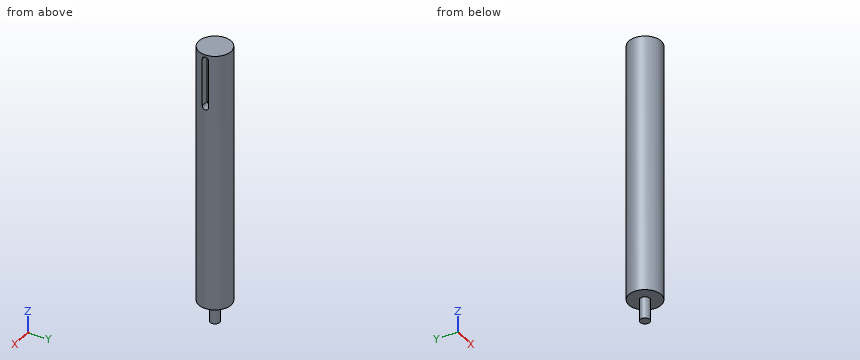
```python
from build123d import *

# Parameters (mm, degrees)
SKETCH_1_R          = 15
EXTRUDE_1_DEPTH     = 240
SKETCH_4_R          = 4.5
EXTRUDE_2_DEPTH     = 20
CUT_EXTRUDE_3_DEPTH = 8


with BuildPart() as part:
    # 草图1 → 凸台-拉伸1 (new body)
    with BuildSketch(Plane.XY):
        Circle(SKETCH_1_R)
    extrude(amount=EXTRUDE_1_DEPTH)

    # 草图4 → 凸台-拉伸2 (add)
    with BuildSketch(Plane(origin=(0, 0, 0), x_dir=(-1, 0, 0), z_dir=(0, 0, -1))):
        Circle(SKETCH_4_R)
    extrude(amount=EXTRUDE_2_DEPTH)

    # 草图5 → 切除-拉伸3 (cut)
    with BuildSketch(Plane(origin=(15, 0, 0), x_dir=(0, 0, -1), z_dir=(1, 0, 0))):
        with BuildLine():
            Line((-235, 3), (-191, 3))
            ThreePointArc((-191, 3), (-188, 0), (-191, -3))
            Line((-191, -3), (-235, -3))
            ThreePointArc((-235, -3), (-238, 0), (-235, 3))
        make_face()
    extrude(amount=-CUT_EXTRUDE_3_DEPTH, mode=Mode.SUBTRACT)


solid = part.part
```
The model under review builds one solid part; all positions refer to its coordinate system, in mm. Round coordinates to 2 decimals unless told otherwise and drop trailing zeros. Write each loop counter-clockwise with the first axis right and the second up, starting at its lowest first coordinate (ties: lowest second). Pieces come first, ordered by that corner, then holes. Notation, with made-up numbers: (-5.75, 35.5) - (38.25, 35.5) arc R17 ccw to (38.25, 66.5) - close; hole circle Ø3 at (-16.5, -39.75). An arc over 180 degrees is marked (long way). One line per question, with ' | ' between items.
Item 1: Add section D-D, the plane z = 224. Give the boundary of the cut face in (x, y).
Resolved:
outline: (7, -3) - (7, 3) - (14.7, 3) arc R15 ccw (long way) to (14.7, -3) - close
Item 2: Add section C-C, the plane y = -8. Give the boundary of the cut face in (x, z).
Resolved:
outline: (-12.69, 0) - (12.69, 0) - (12.69, 240) - (-12.69, 240) - close
Item 3: Add section A-A, the plane x = 0. Give the boundary of the cut face in (y, z), then the cut area to 3 significant figures.
Resolved:
outline: (-15, 0) - (-4.5, 0) - (-4.5, -20) - (4.5, -20) - (4.5, 0) - (15, 0) - (15, 240) - (-15, 240) - close | area: 7,380 mm2
Item 4: For P1, Ø2, axis at y = 10.5, z = 195.5, coming from the +X side; P2, Ø5, axis at x = -10.5, y = -2.5, coming from the -Z side; P3, Ø12, axis at y = 10.5, z = 193, coming from the +X side; P4, Ø3, axis at y = -1.5, z = 127, coming from the -X side, all flat-tipped, find the tip position at first contact; note any pin that passes through.
Resolved:
P1: stops at x = 11.61 | P2: stops at z = 0 | P3: stops at x = 14.31 | P4: stops at x = -15
Item 5: To check wall thickness, follow probe 1 along Z at (x, y) = (7, 12); probe 2 along Y at (x, z) = (0.5, 199.5); probe 3 along Y at (x, z) = (-2, 107.5). State the ranges of each line that lie inside material, in increasing order.
Resolved:
probe 1: z = 0 to 240 | probe 2: y = -14.99 to 14.99 | probe 3: y = -14.87 to 14.87
Item 6: Add section B-B, the plane z = 170. Give the boundary of the cut face in (x, y), then the cut area to 3 significant figures.
Resolved:
outline: circle Ø30 at (0, 0) | area: 707 mm2
